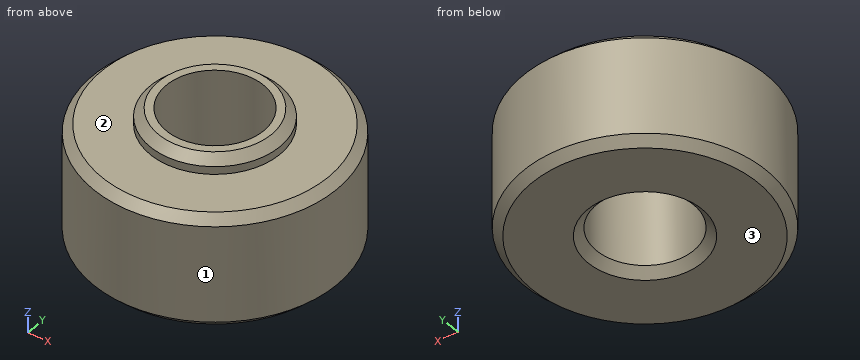
```python
from build123d import *

# Parameters (mm, degrees)
SKETCH1_R           = 7.5
BOSS_EXTRUDE1_DEPTH = 7
SKETCH2_R           = 4
BOSS_EXTRUDE2_DEPTH = 1
SKETCH3_R           = 3
CUT_EXTRUDE1_DEPTH  = 9
CHAMFER1_SIZE       = 0.52


with BuildPart() as part:
    # Sketch1 → Boss-Extrude1 (new body)
    with BuildSketch(Plane.XY):
        Circle(SKETCH1_R)
    extrude(amount=BOSS_EXTRUDE1_DEPTH)

    # Sketch2 → Boss-Extrude2 (add)
    with BuildSketch(Plane.XY.offset(7)):
        Circle(SKETCH2_R)
    extrude(amount=BOSS_EXTRUDE2_DEPTH)

    # Sketch3 → Cut-Extrude1 (cut, through all)
    with BuildSketch(Plane.XY.offset(8)):
        Circle(SKETCH3_R)
    extrude(amount=-CUT_EXTRUDE1_DEPTH, mode=Mode.SUBTRACT)

    # Chamfer1
    chamfer1_edges = [part.edges().sort_by_distance(p)[0] for p in [
        (-3, 0, 0),
        (-7.5, 0, 0),
        (-7.5, 0, 7),
        (-4, 0, 8),
    ]]
    chamfer(chamfer1_edges, length=CHAMFER1_SIZE)


solid = part.part
```
Can you work these out from the model? Positions are in its coordinate system, mm. Face numbers are marked on the shaded views. Give positions to 0.01 mm unless a question says otherwise; leave off trailing zeros. Order: outer loops, then holes, each group sorted by start corner. A loop starts at its lowest first (then second) coordinate and runs counter-clockwise, first axis right, second up. Notation, with made-up numbers: (41.5, 51) - (62.5, 51) arc R9 ccw to (62.5, 65) - close; hole circle Ø10 at (5, 53). An arc over 180 degrees is marked (long way). Use a Markdown table: item, result. Add a question column.
Q1. If we section it at A-A on x = 0: Write out the boundary of the cut face in (y, z).
Q2. If we section it at C-C on z = 5.75: Write out the boundary of the cut face in (x, y).
Q3. If we mould it in two halves opening along Z, with no side actions, what happens to the marked faces 1, 2 and 3? For each: released by +Z, released by -Z, zero draft, split by the parting line, or undercut.
Q4. Please list where these lines run through material, in increasing order: line 1 along Y through (x, z) = (0, 5.75); line 2 along X through (y, z) = (0.25, 2.25); line 3 along Z through (x, y) = (-5.75, 3.25).
Q5. I'm going to push flat-ended pins straight in: pin 1 (1.5 mm diameter, centred on y = 1, z = 3.5, fed in from +X); pin 2 (1.5 mm diameter, centred on x = 5, y = -0.5, fed in from +Z); pin 3 (1.5 mm diameter, centred on x = 1.5, z = 5, fed in from -Y). Where does each tip first touch, or does it pass through?
Answers follow:
| question | item | result |
|---|---|---|
| 1 | outline | (-7.5, 0.52) - (-6.98, 0) - (-3.52, 0) - (-3, 0.52) - (-3, 8) - (-3.48, 8) - (-4, 7.48) - (-4, 7) - (-6.98, 7) - (-7.5, 6.48) - close; (3, 0.52) - (3.52, 0) - (6.98, 0) - (7.5, 0.52) - (7.5, 6.48) - (6.98, 7) - (4, 7) - (4, 7.48) - (3.48, 8) - (3, 8) - close |
| 2 | outline | circle Ø15 at (0, 0); hole circle Ø6 at (0, 0) |
| 3 | face 1 | zero draft |
| 3 | face 2 | released by +Z |
| 3 | face 3 | released by -Z |
| 4 | line 1 | y = -7.5 to -3, 3 to 7.5 |
| 4 | line 2 | x = -7.5 to -2.99, 2.99 to 7.5 |
| 4 | line 3 | z = 0 to 7 |
| 5 | pin 1 | stops at x = 7.5 |
| 5 | pin 2 | stops at z = 7 |
| 5 | pin 3 | stops at y = -7.46 |
